Input: part model. Units: mm. Frame: model coordinates. Face numbers are marked on the shaded views. A direction names the side the tool comes from. Coordinates: 2 decimals unless noted, no trailing zeros. Write each loop counter-clockwise with the first axis right and the second up, starting at its lowest first coordinate (ties: lowest second). Pieces come first, ordered by that corner, then holes. Notation, with made-up numbers: (6.5, 76) - (25.5, 76) arc R18 cw to (25.5, 87) - close; hole circle Ø3 at (60.5, 39.5). An arc over 180 degrees is marked (long way). Use a Markdown table: item, result. Add a question column.
Q1. Section query B-B (y = 0). Return the cut outline in (x, z).
Q2. Material intervals for probe 1 along Y at (x, z) = (-21, 2); probe 2 along Y at (x, z) = (17, 1.5); probe 3 along X at (y, z) = (-26, 2.75), sorted ascending. Write a range as from..to.
Q3. Section query A-A (x = 0). Return the cut outline in (y, z), then the cut area to 3 significant figures.
Q4. Mould query, pull axis X, two halves, no side actions, for the marked faces 3, 4 and 5. Classes: released by +X, released by -X, zero draft, split by the parting line, or undercut.
Q5. Set-up query: the marked faces 1 and 2. Return all of +Z, -Z, +X, -X, +Y, -Y with unobstructed straight access to the full face (end or side cutting, diameter ignored); none if empty.
Q6. Pin query (flat end, axial travel): P1, Ø3, axis at x = 9.5, z = -2, coming from the -Y side; P2, Ø1.5, axis at x = 11, y = 0, coming from the -Z side; P3, Ø1.5, axis at x = -9, z = -5, coming from the -Y side. Return the tip coordinate at first contact, or that it passes through.
Q7. Section query C-C (z = 3.75). Return the cut outline in (x, y), then the cut area to 3 significant figures.
Q8. Section query D-D (y = -27). Return the cut outline in (x, z).
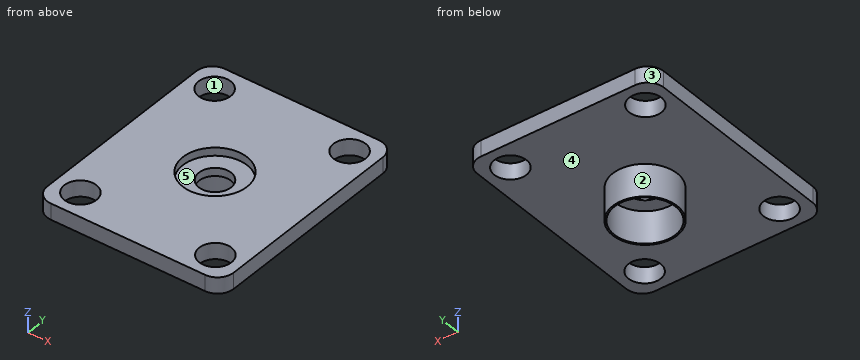
from build123d import *

# Parameters (mm, degrees)
F0_W     = 58
F0_H     = 70
F0_R     = 5
F0_R_2   = 10
F1_DEPTH = 5
F0_R_3   = 9.5
F2_DEPTH = 2.5
F3_DEPTH = 10
F4_R     = 5


with BuildPart() as f1:
    # F0 (on Top) → F1 (new body)
    with BuildSketch(Plane.XY):
        Rectangle(F0_W, F0_H)
        with Locations((-21, -27)):
            Circle(F0_R, mode=Mode.SUBTRACT)
        with Locations((21, -27)):
            Circle(F0_R, mode=Mode.SUBTRACT)
        with Locations((-21, 27)):
            Circle(F0_R, mode=Mode.SUBTRACT)
        Circle(F0_R_2, mode=Mode.SUBTRACT)
        with Locations((21, 27)):
            Circle(F0_R, mode=Mode.SUBTRACT)
    extrude(amount=F1_DEPTH)

    # F0 (on Top) → F2 (join)
    with BuildSketch(Plane.XY):
        Circle(F0_R_2)
        Circle(F0_R_3, mode=Mode.SUBTRACT)
        Circle(F0_R_3)
        Circle(F0_R, mode=Mode.SUBTRACT)
    extrude(amount=F2_DEPTH)

    # F0 (on Top) → F3 (join)
    with BuildSketch(Plane.XY):
        Circle(F0_R_2)
        Circle(F0_R_3, mode=Mode.SUBTRACT)
    extrude(amount=-F3_DEPTH)

    # F4
    f4_edges = [f1.edges().sort_by_distance(p)[0] for p in [
        (-29, -35, 2.5),
        (29, -35, 2.5),
        (29, 35, 2.5),
        (-29, 35, 2.5),
    ]]
    fillet(f4_edges, radius=F4_R)


solid = f1.part
Values follow:
| question | item | result |
|---|---|---|
| 1 | outline | (-29, 0) - (-10, 0) - (-10, -10) - (-9.5, -10) - (-9.5, 0) - (-5, 0) - (-5, 2.5) - (-10, 2.5) - (-10, 5) - (-29, 5) - close; (5, 0) - (9.5, 0) - (9.5, -10) - (10, -10) - (10, 0) - (29, 0) - (29, 5) - (10, 5) - (10, 2.5) - (5, 2.5) - close |
| 2 | probe 1 | -35..-32, -22..22, 32..35 |
| 2 | probe 2 | -35..-30, -24..24, 30..35 |
| 2 | probe 3 | -29..-25.9, -16.1..16.1, 25.9..29 |
| 3 | outline | (-35, 0) - (-10, 0) - (-10, -10) - (-9.5, -10) - (-9.5, 0) - (-5, 0) - (-5, 2.5) - (-10, 2.5) - (-10, 5) - (-35, 5) - close; (5, 0) - (9.5, 0) - (9.5, -10) - (10, -10) - (10, 0) - (35, 0) - (35, 5) - (10, 5) - (10, 2.5) - (5, 2.5) - close |
| 3 | area | 285 mm2 |
| 4 | face 3 | released by -X |
| 4 | face 4 | zero draft |
| 4 | face 5 | undercut |
| 5 | face 1 | +Z, -Z |
| 5 | face 2 | -Z |
| 6 | P1 | y = -6 |
| 6 | P2 | z = 0 |
| 6 | P3 | y = -5.65 |
| 7 | outline | (-29, -30) arc R5 ccw to (-24, -35) - (24, -35) arc R5 ccw to (29, -30) - (29, 30) arc R5 ccw to (24, 35) - (-24, 35) arc R5 ccw to (-29, 30) - close; hole circle Ø10 at (-21, -27); hole circle Ø10 at (-21, 27); hole circle Ø20 at (0, 0); hole circle Ø10 at (21, -27); hole circle Ø10 at (21, 27) |
| 7 | area | 3,410 mm2 |
| 8 | outline | (-29, 0) - (-26, 0) - (-26, 5) - (-29, 5) - close; (-16, 0) - (16, 0) - (16, 5) - (-16, 5) - close; (26, 0) - (29, 0) - (29, 5) - (26, 5) - close |
